Build history of the part. All positions in model axes, mm. A direction names the side the tool comes from. Round coordinates to 2 decimals unless told otherwise and drop trailing zeros. Loops run counter-clockwise (first coordinate to the right, second up) from the corner with the lowest first, then second, coordinate; pieces in that order, holes last. Notation, with made-up numbers: (-18.75, 48) -> (-3.75, 48) arc R28 ccw to (-3.75, 71) -> close; hole circle Ø10 at (79.25, 88). An arc over 180 degrees is marked (long way). Put each result on its own line as item: value. Start each with the question number.
Item 1: Cut at D-D, the plane z = 17. List the corners of the cut face in (x, y).
Item 2: Cut at C-C, the plane z = 4.75. List the corners of the cut face in (x, y).
Item 3: Cut at B-B, the plane y = 24. List the corners of the cut face in (x, z).
Item 4: Drill centre lines: probe 1 along Y at (x, z) = (0, 3.7); probe 2 along Y at (x, z) = (0, 0.8); probe 3 along X at (y, z) = (-18, 9.25). Where is each one in solid material? Low to high. Write a range as [from, to].
Item 5: Flat gauge pins, fed straight in: pin 1 Ø5 at (x, y) = (12, -3.5) entering from +Z; pin 2 Ø4.5 at (y, z) = (-5, 11) entering from +X; pin 3 Ø11.5 at (y, z) = (6.5, 15) entering from -X. Where does each tip first touch, or does it go through?
Item 6: Tool access for faces 4 (the flat face through (15, -7, 11)), 5 (the flat face through (22, -22, 10)), 6 (the cylindrical face through (-0.423, -12.778, 4.021)), 7 (the flat face through (0, -30, 14)), 8 (the cylindrical face through (12.899, -28.274, 11.926)): list every direction of +Z, -Z, +X, -X, +Y, -Y with a clear straight run to the whole face (end or side of a thin tool).
Item 7: Pull direction Z, two halves, no side cores. Call faces 1 (the flat face through (17.47, -1.72, 12.65)), 2 (the flat face through (0, 30, 3)), 3 (the cylindrical face through (-17.101, -28.274, 11.926)): +Z half, -Z half, draft (parallel to the pull), parting line (faces both ways), or undercut.
Item 8: Cut at A-A, the plane x = 0. List the corners of the cut face in (y, z), plus the area to 4 significant figures.
```python
from build123d import *

# Parameters (mm, degrees)
F0_W           = 3
F0_H           = 8
F1_DEPTH       = 20
F0_W_2         = 30
F0_H_2         = 12
F0_H_3         = 40
F0_W_3         = 5
F2_DEPTH       = 5.5
F3_DEPTH       = 20
F5_DEPTH       = 43.001
F7_D           = 3.3
F7_DEPTH       = 13.5002857143
F7_CBORE_D     = 6.5
F7_CBORE_DEPTH = 3
F7_TIP         = 0.9914200214
F8_R           = 5
F9_DEPTH       = 5
F8_R_2         = 2.85
F10_DEPTH      = 3.5
F11_T1_DEPTH   = 30.5
F11_T3_DEPTH   = 33


# Not quite as in the source:
# - a fillet or chamfer that OpenCascade refuses, or shapes differently, is made with other operations: its cross-section is extruded or revolved along the edge and cut away or added


with BuildPart() as f1:
    # F0 (on Top) → F1 (new body)
    with BuildSketch(Plane.XY):
        Polygon((20, -30), (20, -22), (15, -22), (-15, -22), (-20, -22), (-20, -30), align=None)
        with Locations((-21.5, -26)):
            Rectangle(F0_W, F0_H)
        with Locations((21.5, -26)):
            Rectangle(F0_W, F0_H)
    extrude(amount=F1_DEPTH)

    # F0 (on Top) → F2 (join)
    with BuildSketch(Plane.XY):
        with Locations((0, 24)):
            Rectangle(F0_W_2, F0_H_2)
        with Locations((0, -2)):
            Rectangle(F0_W_2, F0_H_3)
        with Locations((-17.5, 24)):
            Rectangle(F0_W_3, F0_H_2)
        with Locations((-17.5, -2)):
            Rectangle(F0_W_3, F0_H_3)
        with Locations((17.5, 24)):
            Rectangle(F0_W_3, F0_H_2)
        with Locations((17.5, -2)):
            Rectangle(F0_W_3, F0_H_3)
    extrude(amount=F2_DEPTH)

    # F0 (on Top) → F3 (join)
    with BuildSketch(Plane.XY):
        with Locations((-17.5, -2)):
            Rectangle(F0_W_3, F0_H_3)
        with Locations((17.5, -2)):
            Rectangle(F0_W_3, F0_H_3)
    extrude(amount=F3_DEPTH)

    # F4 (on face) → F5 (cut, through all)
    with BuildSketch(Plane(origin=(-20, 0, 0), x_dir=(0, -1, 0), z_dir=(-1, 0, 0))):
        Polygon((-18, 20), (-18, 5.5), (22, 20), align=None)
    extrude(amount=-F5_DEPTH, mode=Mode.SUBTRACT)

    # F7
    with Locations(Plane.XY.offset(5.5)):
        with Locations((0, 24), (0, -16)):
            CounterBoreHole(F7_D / 2, F7_CBORE_D / 2, F7_CBORE_DEPTH, depth=F7_DEPTH)
            with Locations((0, 0, -(F7_DEPTH + F7_TIP / 2))):  # 118° drill point
                Cone(0, F7_D / 2, F7_TIP, mode=Mode.SUBTRACT)

    # F8 (on face) → F9 (cut)
    with BuildSketch(Plane.XZ.offset(30)):
        with Locations((0, 7.2906266057)):
            Circle(F8_R)
    extrude(amount=-F9_DEPTH, mode=Mode.SUBTRACT)

    # F8 (on face) → F10 (cut)
    with BuildSketch(Plane.XZ.offset(30)):
        with Locations((-15, 10)):
            Circle(F8_R_2)
        with Locations((15, 10)):
            Circle(F8_R_2)
    extrude(amount=-F10_DEPTH, mode=Mode.SUBTRACT)

    # F11: fillet of radius 5 on 4 edges, made by hand

    # F11_s2 → F11_t1 (cut)
    with BuildSketch(Plane.XY.offset(-12.5)):
        with BuildLine():
            ThreePointArc((15, 30), (18.5355339059, 28.5355339059), (20, 25))
            Line((20, 25), (20, 30))
            Line((20, 30), (15, 30))
        make_face()
        with BuildLine():
            ThreePointArc((-20, 25), (-18.5355339059, 28.5355339059), (-15, 30))
            Line((-15, 30), (-20, 30))
            Line((-20, 30), (-20, 25))
        make_face()
    extrude(amount=F11_T1_DEPTH, mode=Mode.SUBTRACT)

    # F11_s4 → F11_t3 (cut)
    with BuildSketch(Plane.XZ.offset(9.5)):
        with BuildLine():
            ThreePointArc((-23, 15), (-21.5355339059, 18.5355339059), (-18, 20))
            Line((-18, 20), (-23, 20))
            Line((-23, 20), (-23, 15))
        make_face()
        with BuildLine():
            ThreePointArc((18, 20), (21.5355339059, 18.5355339059), (23, 15))
            Line((23, 15), (23, 20))
            Line((23, 20), (18, 20))
        make_face()
    extrude(amount=F11_T3_DEPTH, mode=Mode.SUBTRACT)


solid = f1.part
```
Reply:
1. outline: (-22.58, -30) -> (22.58, -30) -> (22.58, -22) -> (20, -22) -> (20, -13.72) -> (15, -13.72) -> (15, -22) -> (-15, -22) -> (-15, -13.72) -> (-20, -13.72) -> (-20, -22) -> (-22.58, -22) -> close
2. outline: (-23, -30) -> (-4.31, -30) -> (-4.31, -25) -> (4.31, -25) -> (4.31, -30) -> (23, -30) -> (23, -22) -> (20, -22) -> (20, 25) arc R5 ccw to (15, 30) -> (-15, 30) arc R5 ccw to (-20, 25) -> (-20, -22) -> (-23, -22) -> close; hole circle Ø6.5 at (0, -16); hole circle Ø6.5 at (0, 24)
3. outline: (-20, 0) -> (-1.65, 0) -> (-1.65, 2.5) -> (-3.25, 2.5) -> (-3.25, 5.5) -> (-20, 5.5) -> close; (1.65, 0) -> (20, 0) -> (20, 5.5) -> (3.25, 5.5) -> (3.25, 2.5) -> (1.65, 2.5) -> close
4. probe 1: y = [-25, -19.25], [-12.75, 20.75], [27.25, 30]
4. probe 2: y = [-30, -17.65], [-14.35, 22.35], [25.65, 30]
4. probe 3: x = [-20, -15], [15, 20]
5. pin 1: stops at z = 5.5
5. pin 2: stops at x = 20
5. pin 3: stops at x = -20
6. face 4: +Z, +Y
6. face 5: +Z, -Z, +X, +Y
6. face 6: +Z
6. face 7: +Z, -Z, +X, -X, -Y
6. face 8: -Y
7. face 1: +Z half
7. face 2: draft
7. face 3: undercut
8. outline: (-30, 0) -> (-17.65, 0) -> (-17.65, 2.5) -> (-19.25, 2.5) -> (-19.25, 5.5) -> (-22, 5.5) -> (-22, 20) -> (-30, 20) -> (-30, 12.29) -> (-25, 12.29) -> (-25, 2.29) -> (-30, 2.29) -> close; (-14.35, 0) -> (22.35, 0) -> (22.35, 2.5) -> (20.75, 2.5) -> (20.75, 5.5) -> (-12.75, 5.5) -> (-12.75, 2.5) -> (-14.35, 2.5) -> close; (25.65, 0) -> (30, 0) -> (30, 5.5) -> (27.25, 5.5) -> (27.25, 2.5) -> (25.65, 2.5) -> close
8. area: 340.5 mm^2
